Autodesk Inventor part; units mm, degrees
ref_plane "YZ Plane" through (0, 0, 0) normal (1, 0, 0) x (0, 1, 0)
ref_plane "XZ Plane" through (0, 0, 0) normal (0, 1, 0) x (-1, 0, 0)
ref_plane "XY Plane" through (0, 0, 0) normal (0, 0, 1) x (1, 0, 0)
sketch "Sketch1" plane through (0, 0, 0) normal (0, 0, 1) x (1, 0, 0)
  circle A0 centre (0, 0) radius 10
  arc A1 (-28.2843, 14.1421) -> (-14.1421, 28.2843) centre (-21.2132, 21.2132) ccw
  line L0 (-14.1421, 28.2843) -> (-28.706, 42.8482)
  line L1 (-28.2843, 14.1421) -> (-42.8482, 28.706)
  line L2 (50, -20) -> (50, 20)
  arc A2 (-45.9648, 28.3415) -> (49.8462, -20.7692) centre (0, 0) ccw
  arc A3 (49.8462, 20.7692) -> (-28.3415, 45.9648) centre (0, 0) ccw
  arc A4 (-42.8482, 28.706) -> (-45.9648, 28.3415) centre (-44.2624, 27.2918) ccw
  arc A5 (-28.3415, 45.9648) -> (-28.706, 42.8482) centre (-27.2918, 44.2624) ccw
  arc A6 (50, 20) -> (49.8462, 20.7692) centre (48, 20) ccw
  arc A7 (49.8462, -20.7692) -> (50, -20) centre (48, -20) ccw
  line L3 (0, 0) -> (-40.4458, 40.4458) construction
  point P0 (-30.4523, 44.5944)
  point P1 (-44.5944, 30.4523)
  point P2 (50, -20.3961)
  point P3 (50, 20.3961)
  dimension "d1" = 20
  dimension "d4" = 20
  dimension "d12" = 50
  dimension "d13" = 2
  dimension "d14" = 54
  dimension "d15" = 54
  dimension "d16" = 20
  dimension "d19" = 45
  dimension "d21" = 10
  dimension "d22" = 30
extrude "Extrusion3" add sketch "Sketch1" along normal blind 6
properties part number "EndCap 108"
Read the model definition and answer for the solid it produces. Units are mm, in the model's axes. Give positions to 0.01 mm unless a question says otherwise; leave off trailing zeros. Loops run counter-clockwise (first coordinate to the right, second up) from the corner with the lowest first, then second, coordinate; pieces in that order, holes last.
Item 1: The part is cut by section B-B (x = 0). Write down the section's boundary in (y, z).
Item 2: The part is cut by section D-D (y = -17). Write down the section's boundary in (x, z).
Item 3: The mould has two halves that part along X. Classify faces 1 (the flat face through (-35.46, 21.32, 2.96)), 2 (the flat face through (50, 0, 3)), 3 (the flat face through (-3, -11, 0)): released by +X, released by -X, zero draft, split by the parting line, or undercut.
Item 4: The part is cut by section C-C (y = 18). Write down the section's boundary in (x, z), and give its area (3 significant figures).
Item 5: The part is cut by section A-A (z = 2.25). Write down the section's boundary in (x, y).
Item 6: Find the intervals of material crossed by line 1 along Y through (x, z) = (0, 2.05); line 2 along Y through (x, z) = (-18.5, 0.25); line 3 along X through (y, z) = (17, 2.35), in increasing order.
Item 7: Each of these flat-tipped pins is pushed along its axis until it touches: pin 1 Ø1 at (x, z) = (-37, 4.5) entering from +Y; pin 2 Ø1 at (x, y) = (6, 6) entering from -Z; pin 3 Ø2 at (x, z) = (-39, 4) entering from -Y. Where does it stop, or does it pass through?
Taken from the geometry:
1. outline: (-54, 0) - (-10, 0) - (-10, 6) - (-54, 6) - close; (10, 0) - (54, 0) - (54, 6) - (10, 6) - close
2. outline: (-51.25, 0) - (50, 0) - (50, 6) - (-51.25, 6) - close
3. face 1: undercut
3. face 2: released by +X
3. face 3: zero draft
4. outline: (-50.91, 0) - (-32.14, 0) - (-32.14, 6) - (-50.91, 6) - close; (-11.74, 0) - (50, 0) - (50, 6) - (-11.74, 6) - close
4. area: 483 mm2
5. outline: (-45.96, 28.34) arc R54 ccw (long way) to (49.85, -20.77) arc R2 ccw to (50, -20) - (50, 20) arc R2 ccw to (49.85, 20.77) arc R54 ccw to (-28.34, 45.96) arc R2 ccw to (-28.71, 42.85) - (-14.14, 28.28) arc R10 cw to (-28.28, 14.14) - (-42.85, 28.71) arc R2 ccw to start; hole circle Ø20 at (0, 0)
6. line 1: y = -54 to -10, 10 to 54
6. line 2: y = -50.73 to 11.59, 32.64 to 50.73
6. line 3: x = -51.25 to -31.14, -12.14 to 50
7. pin 1: stops at y = 23.36
7. pin 2: passes through
7. pin 3: stops at y = -38.37
